Read the model definition and answer for the solid it produces. Units are mm, in the model's axes. A direction names the side the tool comes from. Round coordinates to 2 decimals unless told otherwise and drop trailing zeros. Write each loop counter-clockwise with the first axis right and the second up, starting at its lowest first coordinate (ties: lowest second). Pieces come first, ordered by that corner, then holes. Notation, with made-up numbers: (61, 27) -> (87, 27) arc R18 ccw to (87, 43) -> close; hole circle Ø10 at (3.25, -32). An arc over 180 degrees is marked (long way). Return JSON: item names as keys, results as strings. Group by question number.
(1) A cutting plane is placed at B-B on y = 0. Give the vertices of the cut face in (x, z), then the cut area to 3 significant figures.
(2) Straight lines are drawn through the part: line 1 (Z direction, x = -2.5, y = 2.25); line 2 (Z direction, x = 0.25, y = 0.75); line 3 (X direction, y = -0.25, z = 1.25). For each, find the intervals that lie inside material, in ascending order.
(3) For faces 4 (the cylindrical face through (0, -2, -6)), 5 (the flat face through (-0.64, 1.13, 2.03)), 6 (the flat face through (0, 0, -12)), determine the directions among +Z, -Z, +X, -X, +Y, -Y from which every point of the face is accessible in a straight line to the end or side of a thin tool.
(4) A cutting plane is placed at C-C on x = 0.25. Give the vertices of the cut face in (y, z).
(5) Given pin 1 (3 mm diameter, centred on x = -0.5, y = 0.5, fed in from +Z); pin 2 (2 mm diameter, centred on y = 1, z = -10, fed in from +X), each flat-ended and moving along its own axis, determine where each tip first touches the part or whether it passes through.
(6) A cutting plane is placed at A-A on z = 1.5. Give the vertices of the cut face in (x, y), then the cut area to 3 significant figures.
(7) A cutting plane is placed at D-D on z = -9. Give the vertices of the cut face in (x, y), then the cut area to 3 significant figures.
(8) The mould has two halves that part along X. Classify faces 1 (the cylindrical face through (3.233, -1.341, 1.972)), 2 (the flat face through (2, -2, 0)), 3 (the flat face through (0.66, 1.12, 2.03)): released by +X, released by -X, zero draft, split by the parting line, or undercut.
```python
from build123d import *

# Parameters (mm, degrees)
F0_R     = 3.5
F0_R_2   = 2
F1_DEPTH = 4
F2_DEPTH = 12
F4_DEPTH = 4


with BuildPart() as f1:
    # F0 (on Top) → F1 (new body)
    with BuildSketch(Plane.XY):
        Circle(F0_R)
        Circle(F0_R_2, mode=Mode.SUBTRACT)
        Circle(F0_R_2)
    extrude(amount=F1_DEPTH)

    # F0 (on Top) → F2 (join)
    with BuildSketch(Plane.XY):
        Circle(F0_R_2)
    extrude(amount=-F2_DEPTH)

    # F3 (on face) → F4 (cut, through all)
    with BuildSketch(Plane.XY.offset(4)):
        Polygon((-1.299038, -0.75), (0, -1.5), (1.299038, -0.75), (1.299038, 0.75), (0, 1.5), (-1.299038, 0.75), align=None)
    extrude(amount=-F4_DEPTH, mode=Mode.SUBTRACT)


solid = f1.part
```
Checks:
{
 "1": {"outline": "(-3.5, 0) -> (-2, 0) -> (-2, -12) -> (2, -12) -> (2, 0) -> (3.5, 0) -> (3.5, 4) -> (1.3, 4) -> (1.3, 0) -> (-1.3, 0) -> (-1.3, 4) -> (-3.5, 4) -> close", "area": "65.6 mm^2"},
 "2": {"line 1": "z = 0 to 4", "line 2": "z = -12 to 0", "line 3": "x = -3.49 to -1.3, 1.3 to 3.49"},
 "3": {"face 4": "-Z", "face 5": "+Z", "face 6": "-Z, +X, -X, +Y, -Y"},
 "4": {"outline": "(-3.49, 0) -> (-1.98, 0) -> (-1.98, -12) -> (1.98, -12) -> (1.98, 0) -> (3.49, 0) -> (3.49, 4) -> (1.36, 4) -> (1.36, 0) -> (-1.36, 0) -> (-1.36, 4) -> (-3.49, 4) -> close"},
 "5": {"pin 1": "stops at z = 4", "pin 2": "stops at x = 2"},
 "6": {"outline": "circle Ø7 at (0, 0); hole (-1.3, -0.75) -> (0, -1.5) -> (1.3, -0.75) -> (1.3, 0.75) -> (0, 1.5) -> (-1.3, 0.75) -> close", "area": "32.6 mm^2"},
 "7": {"outline": "circle Ø4 at (0, 0)", "area": "12.6 mm^2"},
 "8": {"face 1": "split by the parting line", "face 2": "zero draft", "face 3": "undercut"}
}
